from build123d import *

# Parameters (mm, degrees)
BOSS_EXTRUDE1_DEPTH = 12.7
SKETCH2_R           = 3.3782
CUT_EXTRUDE1_DEPTH  = 486.307863629
FILLET1_R           = 6.35
SKETCH4_R           = 3.937
CUT_EXTRUDE2_DEPTH  = 486.307863629


with BuildPart() as part:
    # Sketch1 → Boss-Extrude1 (new body)
    with BuildSketch(Plane.XY):
        with BuildLine():
            Line((63.5, 0), (63.5, 120.65))
            Line((63.5, 120.65), (458.219565432, 88.85900811))
            ThreePointArc((458.219565432, 88.85900811), (466.533768826, 84.812244743), (469.9, 76.2))
            Line((469.9, 76.2), (469.9, 0))
            Line((469.9, 0), (63.5, 0))
        make_face()
    extrude(amount=BOSS_EXTRUDE1_DEPTH)

    # Sketch2 → Cut-Extrude1 (cut, through all)
    with BuildSketch(Plane.XY.offset(12.7)):
        with Locations((127, 12.7)):
            Circle(SKETCH2_R)
        with Locations((381, 12.7)):
            Circle(SKETCH2_R)
    extrude(amount=-CUT_EXTRUDE1_DEPTH, mode=Mode.SUBTRACT)

    # Fillet1
    fillet1_edges = [part.edges().sort_by_distance(p)[0] for p in [
        (469.9, 0, 6.35),
    ]]
    fillet(fillet1_edges, radius=FILLET1_R)

    # Sketch4 → Cut-Extrude2 (cut, through all)
    with BuildSketch(Plane(origin=(0, 0, 0), x_dir=(-1, 0, 0), z_dir=(0, 0, -1))):
        with Locations((-416.56762, 76.2)):
            Circle(SKETCH4_R)
        with Locations((-416.56762, 19.05)):
            Circle(SKETCH4_R)
    extrude(amount=-CUT_EXTRUDE2_DEPTH, mode=Mode.SUBTRACT)


solid = part.part
Design review of the part built by this model. Coordinates are the model's own, in mm. Coordinates: 2 decimals unless noted, no trailing zeros. Write each loop counter-clockwise with the first axis right and the second up, starting at its lowest first coordinate (ties: lowest second). Pieces come first, ordered by that corner, then holes. Notation, with made-up numbers: (-27, -15.75) - (14, -15.75) arc R13 ccw to (14, -11.75) - close; hole circle Ø5 at (8.25, -21.75). An arc over 180 degrees is marked (long way). Use one line per item in the form item = value.
Q1. Consider section B-B (x = 343.5). Write out the cut boundary in (y, z), plus the area to 3 significant figures.
Taken from the geometry:
outline = (0, 0) - (98.1, 0) - (98.1, 12.7) - (0, 12.7) - close
area = 1,250 mm^2
Q2. Consider section A-A (z = 5). Write out the cut boundary in (x, y), plus the area to 3 significant figures.
Taken from the geometry:
outline = (63.5, 0) - (463.55, 0) arc R6.35 ccw to (469.9, 6.35) - (469.9, 76.2) arc R12.7 ccw to (458.22, 88.86) - (63.5, 120.65) - close; hole circle Ø6.76 at (127, 12.7); hole circle Ø6.76 at (381, 12.7); hole circle Ø7.87 at (416.57, 19.05); hole circle Ø7.87 at (416.57, 76.2)
area = 42,200 mm^2
Q3. For probe 1 along Y at (x, z) = (127, 8.25); probe 2 along X at (y, z) = (78, 8.5); probe 3 along Y at (x, z) = (381, 9.25), list the stretches that pass through material, from the lowest coordinate up.
Taken from the geometry:
probe_1 = 0 to 9.32, 16.08 to 115.54
probe_2 = 63.5 to 413.07, 420.07 to 469.77
probe_3 = 0 to 9.32, 16.08 to 95.08
Q4. Insertion check: pin 1 Ø9 at (x, y) = (127, 12.7) entering from -Z; pin 2 Ø5 at (y, z) = (86.5, 10.5) entering from +X; pin 3 Ø6.5 at (x, y) = (416.57, 76.2) entering from -Z. Each pin has a flat end and moves straight along its axis. Give the tip position at first contact, or say it passes through.
Taken from the geometry:
pin_1 = 0
pin_2 = 467.22
pin_3 = through
Q5. Consider section C-C (x = 440.5). Write out the cut boundary in (y, z).
Taken from the geometry:
outline = (0, 0) - (90.29, 0) - (90.29, 12.7) - (0, 12.7) - close
Q6. The part is to be moulded in two halves that separate along X. For faces 1 (the cylindrical face through (377.625, 12.849, 6.439)), 2 (the flat face through (270, 48, 0)), 3 (the cylindrical face through (420.5, 76.4, 6.3)), 4 (the cylindrical face through (466.44, 84.91, 6.26)), say which applies: +X half, -X half, draft (parallel to the pull), parting line (faces both ways), or undercut.
Taken from the geometry:
face_1 = undercut
face_2 = draft
face_3 = undercut
face_4 = +X half
